For this review, use the dimensioned drawing (mm, ordinates from the lowest corner) and the shaded views. Round coordinates to 2 decimals unless told otherwise and drop trailing zeros. Write each loop counter-clockwise with the first axis right and the second up, starting at its lowest first coordinate (ties: lowest second). Pieces come first, ordered by that corner, then holes. Notation, with made-up numbers: M -5,70.5 L 8,70.5 A12 ccw 8,85.5 Z; hole C -26.5,-28 d5. An arc over 180 degrees is marked long. One line per question, with ' | ' between items.
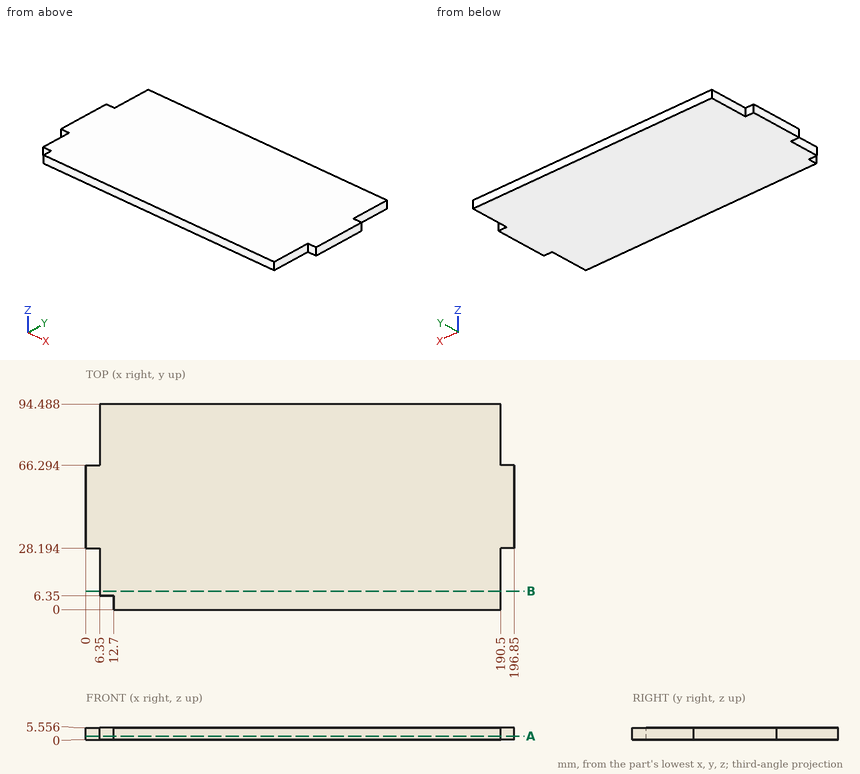
Item 1: To check wall thickness, follow line 1 along X through (y, z) = (88, 0.55); line 2 along X through (y, z) = (4.5, 0.3). State the ranges of each line that lie inside material, in increasing order. Write a range as from..to.
Results:
line 1: 6.35..190.5 | line 2: 12.7..190.5
Item 2: Insertion check: pin 1 Ø3 at (y, z) = (21, 3) entering from +X; pin 2 Ø1.7 at (y, z) = (2, 1.5) entering from -X; pin 3 Ø3 at (x, z) = (3.5, 2.5) entering from +Y. Each pin has a flat end and moves straight along its axis. Give the tip position at first contact, or say it passes through.
Results:
pin 1: x = 190.5 | pin 2: x = 12.7 | pin 3: y = 66.29
Item 3: Take a section at B-B (y = 8.5). Write out the cut boundary in (x, z), then the cut area to 3 significant figures.
Results:
outline: M 6.35,0 L 190.5,0 L 190.5,5.56 L 6.35,5.56 Z | area: 1,020 mm2
Item 4: Take a section at A-A (z = 1.6). Write out the cut boundary in (x, y), then the cut area to 3 significant figures.
Results:
outline: M 0,28.19 L 6.35,28.19 L 6.35,6.35 L 12.7,6.35 L 12.7,0 L 190.5,0 L 190.5,28.19 L 196.85,28.19 L 196.85,66.29 L 190.5,66.29 L 190.5,94.49 L 6.35,94.49 L 6.35,66.29 L 0,66.29 Z | area: 17,800 mm2
